Can you work these out from the model? Positions are in its coordinate system, mm. Face numbers are marked on the shaded views. A direction names the side the tool comes from. Give positions to 0.01 mm unless a question says otherwise; leave off trailing zeros. Loops run counter-clockwise (first coordinate to the right, second up) from the corner with the lowest first, then second, coordinate; pieces in that order, holes last. Notation, with made-up numbers: (32, 44) - (44, 44) arc R18 cw to (44, 69) - close; hole circle Ø7 at (72, 78.5). An arc over 180 degrees is marked (long way). Write item = value, one per line.
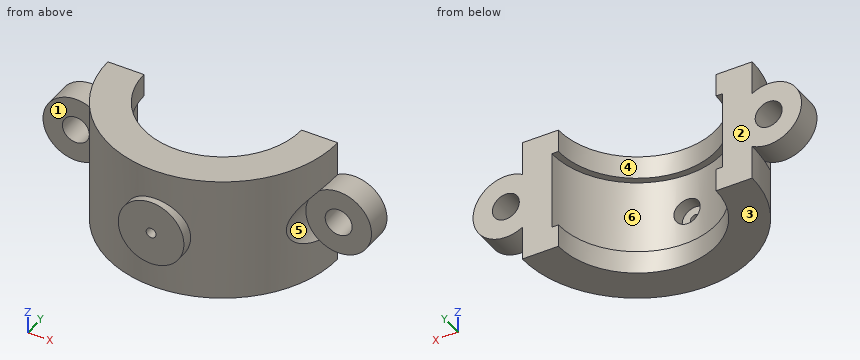
from build123d import *

# Parameters (mm, degrees)
EXTRUDE_2_DEPTH     = 19
SKETCH_2_R          = 10
EXTRUDE_3_DEPTH     = 40
SKETCH_3_R          = 10
CUT_EXTRUDE_1_DEPTH = 32
SKETCH_4_R          = 4.1
CUT_EXTRUDE_2_DEPTH = 9.0000001
EXTRUDE_START       = -37
SKETCH_5_R          = 10
SKETCH_5_R_2        = 1.5
EXTRUDE_4_DEPTH     = 3.45898
SKETCH_5_4_R        = 1.5
CUT_EXTRUDE_3_DEPTH = 38.0000001
CUT_EXTRUDE_4_DEPTH = 12
SKETCH_6_R          = 4
CUT_EXTRUDE_5_DEPTH = 30


with BuildPart() as part:
    # Эскиз1 → Бобышка-Вытянуть2 (new body, symmetric)
    with BuildSketch(Plane.XY):
        with BuildLine():
            Line((35, 0), (26, 0))
            ThreePointArc((26, 0), (0, -26), (-26, 0))
            Line((-26, 0), (-35, 0))
            ThreePointArc((-35, 0), (0, -35), (35, 0))
        make_face()
        with BuildLine():
            Line((26, 0), (24, 0))
            ThreePointArc((24, 0), (0, -24), (-24, 0))
            Line((-24, 0), (-26, 0))
            ThreePointArc((-26, 0), (0, -26), (26, 0))
        make_face()
    extrude(amount=EXTRUDE_2_DEPTH, both=True)

    # Эскиз2 → Бобышка-Вытянуть3 (add)
    with BuildSketch(Plane(origin=(0, 0, 0), x_dir=(1, 0, 0), z_dir=(0, 1, 0))):
        with Locations((40, 0)):
            Circle(SKETCH_2_R)
    extrude_3 = extrude(amount=-EXTRUDE_3_DEPTH)

    # Эскиз3 → Вырез-Вытянуть1 (cut)
    with BuildSketch(Plane.XZ.offset(40)):
        with Locations((40, 0)):
            Circle(SKETCH_3_R)
    cut_extrude_1 = extrude(amount=-CUT_EXTRUDE_1_DEPTH, mode=Mode.SUBTRACT)

    # Эскиз4 → Вырез-Вытянуть2 (cut, through all)
    with BuildSketch(Plane.XZ.offset(8)):
        with Locations((40, 0)):
            Circle(SKETCH_4_R)
    cut_extrude_2 = extrude(amount=-CUT_EXTRUDE_2_DEPTH, mode=Mode.SUBTRACT)

    # Зеркальное отражение1: Бобышка-Вытянуть3, Вырез-Вытянуть1, Вырез-Вытянуть2 across plane
    add(extrude_3.mirror(Plane(origin=(0, 0, 0), x_dir=(0, 0, 1), z_dir=(1, 0, 0))))
    add(cut_extrude_1.mirror(Plane(origin=(0, 0, 0), x_dir=(0, 0, 1), z_dir=(1, 0, 0))), mode=Mode.SUBTRACT)
    add(cut_extrude_2.mirror(Plane(origin=(0, 0, 0), x_dir=(0, 0, 1), z_dir=(1, 0, 0))), mode=Mode.SUBTRACT)

    # Эскиз5 → Бобышка-Вытянуть4 (add)
    with BuildSketch(Plane(origin=(0, 0, 0), x_dir=(1, 0, 0), z_dir=(0, 1, 0)).offset(EXTRUDE_START)):
        Circle(SKETCH_5_R)
        Circle(SKETCH_5_R_2, mode=Mode.SUBTRACT)
        Circle(SKETCH_5_R_2)
    extrude(amount=EXTRUDE_4_DEPTH)

    # Эскиз5<4> → Вырез-Вытянуть3 (cut, through all)
    with BuildSketch(Plane(origin=(0, 0, 0), x_dir=(1, 0, 0), z_dir=(0, 1, 0))):
        Circle(SKETCH_5_4_R)
    extrude(amount=-CUT_EXTRUDE_3_DEPTH, mode=Mode.SUBTRACT)

    # Эскиз1<4> → Вырез-Вытянуть4 (cut, symmetric)
    with BuildSketch(Plane.XY):
        with BuildLine():
            ThreePointArc((-24, 0), (0, 24), (24, 0))
            Line((24, 0), (26, 0))
            ThreePointArc((26, 0), (0, 26), (-26, 0))
            Line((-26, 0), (-24, 0))
        make_face()
        with BuildLine():
            Line((26, 0), (24, 0))
            ThreePointArc((24, 0), (0, -24), (-24, 0))
            Line((-24, 0), (-26, 0))
            ThreePointArc((-26, 0), (0, -26), (26, 0))
        make_face()
    extrude(amount=CUT_EXTRUDE_4_DEPTH, both=True, mode=Mode.SUBTRACT)

    # Эскиз6 → Вырез-Вытянуть5 (cut)
    with BuildSketch(Plane(origin=(0, 0, 0), x_dir=(1, 0, 0), z_dir=(0, 1, 0))):
        Circle(SKETCH_6_R)
    extrude(amount=-CUT_EXTRUDE_5_DEPTH, mode=Mode.SUBTRACT)


solid = part.part
Q1. For pin 1 (2.5 mm diameter, centred on x = 2, z = -2, fed in from +Y); pin 2 (4 mm diameter, centred on x = -18.5, z = -10.5, fed in from -Y); pin 3 (16 mm diameter, centred on x = -44, z = -3.5, fed in from -Y), each with a flat end and sliding along its axis, tell me the tip position at first contact or that it passes through.
Output:
pin_1 = -25.81
pin_2 = -30.87
pin_3 = -8
Q2. Which directions (+Z, -Z, +X, -X, +Y, -Y) give clear straight access to the entire face, cutting with the end or side of a thin tool? Please do the marked faces 4, 5 and 6.
Output:
face_4 = +Z, -Z, +Y
face_5 = +X, -Y
face_6 = +Y
Q3. I need wall thicknesses on L1, parallel to Z at x = -40, y = -6; L2, parallel to Z at x = 0, y = -27.9; L3, parallel to X at y = -4, z = 0.5. Which ranges of each line are inside material? Lowest first, please.
Output:
L1 = -10 to -4.1, 4.1 to 10
L2 = -19 to -4, 4 to 19
L3 = -49.99 to -44.07, -35.93 to -25.69, 25.69 to 35.93, 44.07 to 49.99
Q4. Imagine slicing it at A-A, the plane x = 0. Write out the boundary of the cut face in (y, z), then the cut area to 3 significant figures.
Output:
outline = (-37, -10) - (-35, -10) - (-35, -19) - (-24, -19) - (-24, -12) - (-26, -12) - (-26, -4) - (-30, -4) - (-30, -1.5) - (-37, -1.5) - close; (-37, 1.5) - (-30, 1.5) - (-30, 4) - (-26, 4) - (-26, 12) - (-24, 12) - (-24, 19) - (-35, 19) - (-35, 10) - (-37, 10) - close
area = 357 mm2
Q5. Imagine slicing it at D-D, the plane x = -40. Write out the boundary of the cut face in (y, z), then the cut area to 3 significant figures.
Output:
outline = (-8, -10) - (0, -10) - (0, -4.1) - (-8, -4.1) - close; (-8, 4.1) - (0, 4.1) - (0, 10) - (-8, 10) - close
area = 94.4 mm2
Q6. We'd pull the mould along Z, two halves only. Please class the marked faces 1, 2 and 3: released by +Z, released by -Z, zero draft, split by the parting line, or undercut.
Output:
face_1 = undercut
face_2 = zero draft
face_3 = released by -Z
Q7. Imagine slicing it at C-C, the plane z = 2.5. Write out the boundary of the cut face in (x, y), then the cut area to 3 significant figures.
Output:
outline = (-49.68, -8) - (-43.25, -8) - (-43.25, 0) - (-49.68, 0) - close; (-36.75, -8) - (-30.32, -8) - (-30.32, -17.49) arc R35 ccw to (-9.68, -33.63) - (-9.68, -37) - (9.68, -37) - (9.68, -33.63) arc R35 ccw to (30.32, -17.49) - (30.32, -8) - (36.75, -8) - (36.75, 0) - (26, 0) arc R26 cw to (3.12, -25.81) - (3.12, -30) - (-3.12, -30) - (-3.12, -25.81) arc R26 cw to (-26, 0) - (-36.75, 0) - close; (43.25, -8) - (49.68, -8) - (49.68, 0) - (43.25, 0) - close
area = 980 mm2
Q8. Imagine slicing it at B-B, the plane y = -9. Write out the boundary of the cut face in (x, z), then the cut area to 3 significant figures.
Output:
outline = (-33.82, -19) - (-22.25, -19) - (-22.25, -12) - (-24.39, -12) - (-24.39, 12) - (-22.25, 12) - (-22.25, 19) - (-33.82, 19) - (-33.82, 7.86) arc R10 cw to (-33.82, -7.86) - close; (22.25, -19) - (33.82, -19) - (33.82, -7.86) arc R10 cw to (33.82, 7.86) - (33.82, 19) - (22.25, 19) - (22.25, 12) - (24.39, 12) - (24.39, -12) - (22.25, -12) - close
area = 693 mm2
